from build123d import *

# Parameters (mm, degrees)
SKETCH1_R           = 2.5
BOSS_EXTRUDE1_DEPTH = 25
FILLET1_R           = 1
FILLET2_R           = 0.5
FILLET3_R           = 0.5
FILLET4_R           = 0.5
FILLET5_R           = 0.5


with BuildPart() as part:
    # Sketch1 → Boss-Extrude1 (new, symmetric)
    with BuildSketch(Plane.XY):
        Polygon((13.2, 0), (13.2, 1.8), (15.45, 1.8), (15.45, 3.6), (12.95, 6.1), (7.05, 6.1), (4.55, 3.6), (4.55, 1.8), (6.8, 1.8), (6.8, 0), (0, 0), (0, 6.8), (1.8, 6.8), (1.8, 4.55), (3.6, 4.55), (6.1, 7.05), (6.1, 12.95), (3.6, 15.45), (1.8, 15.45), (1.8, 13.2), (0, 13.2), (0, 20), (6.8, 20), (6.8, 18.2), (4.55, 18.2), (4.55, 16.4), (7.05, 13.9), (12.95, 13.9), (15.45, 16.4), (15.45, 18.2), (13.2, 18.2), (13.2, 20), (20, 20), (20, 13.2), (18.2, 13.2), (18.2, 15.45), (16.4, 15.45), (13.9, 12.95), (13.9, 7.05), (16.4, 4.55), (18.2, 4.55), (18.2, 6.8), (20, 6.8), (20, 0), align=None)
        with Locations((10, 10)):
            Circle(SKETCH1_R, mode=Mode.SUBTRACT)
    extrude(amount=BOSS_EXTRUDE1_DEPTH, both=True)

    # Fillet1
    fillet1_edges = [part.edges().sort_by_distance(p)[0] for p in [
        (0, 0, 0),
        (0, 20, 0),
        (20, 20, 0),
        (20, 0, 0),
    ]]
    fillet(fillet1_edges, radius=FILLET1_R)

    # Fillet2
    fillet2_edges = [part.edges().sort_by_distance(p)[0] for p in [
        (4.55, 18.2, 0),
        (4.55, 16.4, 0),
        (7.05, 13.9, 0),
        (12.95, 13.9, 0),
        (15.45, 16.4, 0),
        (15.45, 18.2, 0),
    ]]
    fillet(fillet2_edges, radius=FILLET2_R)

    # Fillet3
    fillet3_edges = [part.edges().sort_by_distance(p)[0] for p in [
        (18.2, 15.45, 0),
        (16.4, 15.45, 0),
        (13.9, 12.95, 0),
        (13.9, 7.05, 0),
        (16.4, 4.55, 0),
        (18.2, 4.55, 0),
    ]]
    fillet(fillet3_edges, radius=FILLET3_R)

    # Fillet4
    fillet4_edges = [part.edges().sort_by_distance(p)[0] for p in [
        (1.8, 4.55, 0),
        (3.6, 4.55, 0),
        (6.1, 7.05, 0),
        (6.1, 12.95, 0),
        (3.6, 15.45, 0),
        (1.8, 15.45, 0),
    ]]
    fillet(fillet4_edges, radius=FILLET4_R)

    # Fillet5
    fillet5_edges = [part.edges().sort_by_distance(p)[0] for p in [
        (15.45, 1.8, 0),
        (15.45, 3.6, 0),
        (12.95, 6.1, 0),
        (7.05, 6.1, 0),
        (4.55, 3.6, 0),
        (4.55, 1.8, 0),
    ]]
    fillet(fillet5_edges, radius=FILLET5_R)


solid = part.part
Model file for the job. Use its own axes, mm. A direction names the side the tool comes from. Give positions to 0.01 mm unless a question says otherwise; leave off trailing zeros. Loops run counter-clockwise (first coordinate to the right, second up) from the corner with the lowest first, then second, coordinate; pieces in that order, holes last.
Item 1: Slice it at B-B (y = 10). Write the cut outline in (x, z), plus the area to 3 significant figures.
Check values:
outline: (6.1, -25) - (7.5, -25) - (7.5, 25) - (6.1, 25) - close; (12.5, -25) - (13.9, -25) - (13.9, 25) - (12.5, 25) - close
area: 140 mm2
Item 2: Drop flat-ended pins along their axis: P1, Ø6, axis at x = 10, z = 11, coming from the +Y side; P2, Ø2.5, axis at x = 11, z = -9.5, coming from the -Y side; P3, Ø1, axis at y = 11, z = -15.5, coming from the -X side; P4, Ø2, axis at x = 10, y = 9.5, coming from the +Z side. Give the stop position or say it passes through.
Check values:
P1: stops at y = 13.97
P2: stops at y = 6.1
P3: stops at x = 6.1
P4: passes through
Item 3: Drill centre lines: line 1 along Y through (x, z) = (10, 9); line 2 along Y through (x, z) = (3.75, -4); line 3 along X through (y, z) = (1.5, -16). Where is each one in solid material? Low to high.
Check values:
line 1: y = 6.1 to 7.5, 12.5 to 13.9
line 2: y = 0 to 4.7, 15.3 to 20
line 3: x = 0 to 6.8, 13.2 to 20
Item 4: Which spindle directions (+Z, -Z, +X, -X, +Y, -Y) get a long thin tool onto all of the face, cutting with end or side? Do faces 4 (the face through (13.9, 10, 0)), 5 (the face through (10, 6.1, 0)), 6 (the face through (5.82, 4.87, 0.35)), 7 (the face through (6.1, 10, 0)), 8 (the face through (13.2, 19, 0)). Say none if no direction does.
Check values:
face 4: +Z, -Z, +X
face 5: +Z, -Z, -Y
face 6: +Z, -Z
face 7: +Z, -Z, -X
face 8: +Z, -Z, +Y
Item 5: Slice it at A-A (x = 8). Write the cut outline in (y, z), plus the area to 3 significant figures.
Check values:
outline: (6.1, -25) - (8.5, -25) - (8.5, 25) - (6.1, 25) - close; (11.5, -25) - (13.9, -25) - (13.9, 25) - (11.5, 25) - close
area: 240 mm2
Item 6: Mould opens along X. For faces 1 (the face through (19, 6.8, 0)), 2 (the face through (0.301, 19.715, -0.35)), 3 (the face through (14.22, 4.83, 0.35)) say: +X half, -X half, draft (parallel to the pull), parting line (faces both ways), or undercut.
Check values:
face 1: draft
face 2: -X half
face 3: undercut
